from build123d import *

# Parameters (mm, degrees)
MODEL_R         = 19.166698656
MODEL_R_2       = 18.385271544
MODEL_R_3       = 16.640009412
MODEL_R_4       = 16.752801617
MODEL_W         = 2
MODEL_H         = 10
MODEL_W_2       = 2.0625
MODEL_W_3       = 5
MODEL_H_2       = 5
EXTRUDE_1_DEPTH = 1.5


with BuildPart() as part:
    # Model → 凸台-拉伸1 (new body)
    with BuildSketch(Plane.XY):
        Polygon((331.008501053, -12.681071835), (341.616416104, -12.681071835), (341.616416104, -14.681071835), (346.616416104, -14.681071835), (346.616416104, -12.681071835), (359.731458438, -12.681071835), (359.731458438, -14.681071835), (364.731458438, -14.681071835), (364.731458438, -12.681071835), (389.285051542, -12.681071835), (389.285051542, -14.681071835), (394.285051542, -14.681071835), (394.285051542, -12.681071835), (438.527315214, -12.681071835), (438.527315214, -13.681071835), (443.527315214, -13.681071835), (443.527315214, -12.681071835), (466.595113664, -12.681071835), (466.595113664, -13.681071835), (471.595113664, -13.681071835), (471.595113664, -12.681071835), (509.543834164, -12.681071835), (509.543834164, -13.681071835), (514.543834164, -13.681071835), (514.543834164, -12.681071835), (534.941100783, -12.681071835), (534.941100783, -13.681071835), (539.941100783, -13.681071835), (539.941100783, -12.681071835), (567.393171936, -12.681071835), (567.393171936, -13.681071835), (572.393171936, -13.681071835), (572.393171936, -12.681071835), (590.909160047, -12.681071835), (590.909160047, -13.681071835), (595.909160047, -13.681071835), (595.909160047, -12.681071835), (621.009616189, -12.681071835), (621.009616189, -14.681071835), (626.009616189, -14.681071835), (626.009616189, -12.681071835), (639.352091775, -12.681071835), (639.352091775, -14.681071835), (644.352091775, -14.681071835), (644.352091775, -12.681071835), (662.203652971, -12.681071835), (662.203652971, -14.681071835), (667.203652971, -14.681071835), (667.203652971, -12.681071835), (673.375169904, -12.681071835), (673.375169904, 40.318928165), (667.203652971, 40.318928165), (667.203652971, 41.318928165), (662.203652971, 41.318928165), (662.203652971, 40.318928165), (619.461197001, 40.318928165), (618.879989346, 40.463263521), (612.469969479, 41.955284735), (606.036780234, 43.352226087), (599.689619006, 44.633304674), (593.327411645, 45.82195159), (586.94928996, 46.921207599), (580.557470145, 47.935980702), (574.151952199, 48.866270901), (567.734908698, 49.715987149), (561.30547145, 50.48817021), (554.907598578, 51.180900831), (548.503413488, 51.797834645), (542.093915228, 52.338928034), (535.680059227, 52.803138329), (529.259803769, 53.18955372), (522.834147903, 53.498130589), (516.404003437, 53.72682722), (509.962377034, 53.875948948), (503.521170035, 53.942974245), (497.0802952, 53.925905013), (490.639752529, 53.824741253), (488.943859674, 53.774868005), (488.943859674, 48.550761193), (490.943859674, 48.550761193), (490.943859674, 38.550761193), (488.943859674, 38.550761193), (488.943859674, 44.701347368), (483.943859674, 44.701347368), (483.943859674, 38.550761193), (481.943859674, 38.550761193), (481.943859674, 48.550761193), (483.943859674, 48.550761193), (483.943859674, 53.624339658), (477.764179108, 53.358922521), (471.328973881, 52.990271357), (464.822470484, 52.524637869), (458.325635443, 51.959487936), (451.839336947, 51.291780793), (445.366397665, 50.51738939), (438.908510356, 49.62923315), (432.467542259, 48.62422769), (426.046316041, 47.498245959), (422.774988305, 46.874345456), (419.510213514, 46.217127406), (416.253034336, 45.527547239), (413.004318963, 44.80256419), (409.762156535, 44.044263594), (406.528457911, 43.250560117), (403.303179471, 42.420454711), (400.000268013, 41.531679768), (396.709598454, 40.602332225), (395.753608128, 40.318928165), (364.731458438, 40.318928165), (364.731458438, 41.318928165), (359.731458438, 41.318928165), (359.731458438, 40.318928165), (346.616416104, 40.318928165), (346.616416104, 41.318928165), (341.616416104, 41.318928165), (341.616416104, 40.318928165), (331.008501053, 40.318928165), align=None)
        with Locations((453.628632303, 20.416282665)):
            Circle(MODEL_R, mode=Mode.SUBTRACT)
        with Locations((517.796175226, 21.864038252)):
            Circle(MODEL_R_2, mode=Mode.SUBTRACT)
        with Locations((576.99591729, 16.073011283)):
            Circle(MODEL_R_3, mode=Mode.SUBTRACT)
        with Locations((378.89019282, 16.048912753)):
            Circle(MODEL_R_4, mode=Mode.SUBTRACT)
        Polygon((334.054616565, 0.346826696), (335.34950157, 3.052981316), (338.055656189, 1.758096311), (336.760771185, -0.948058308), align=None, mode=Mode.SUBTRACT)
        Polygon((488.943859674, 7.212935553), (483.943859674, 7.212935553), (483.943859674, 3.001809248), (481.943859674, 3.001809248), (481.943859674, -6.998190752), (483.943859674, -6.998190752), (483.943859674, -1.850844057), (488.943859674, -1.850844057), (488.943859674, -6.998190752), (490.943859674, -6.998190752), (490.943859674, 3.001809248), (488.943859674, 3.001809248), align=None, mode=Mode.SUBTRACT)
        with Locations((418.104897365, 1.876528165)):
            Rectangle(MODEL_W, MODEL_H, mode=Mode.SUBTRACT)
        with Locations((547.437658193, 3.401778165)):
            Rectangle(MODEL_W, MODEL_H, mode=Mode.SUBTRACT)
        with Locations((603.344317775, 1.378728165)):
            Rectangle(MODEL_W_2, MODEL_H, mode=Mode.SUBTRACT)
        with Locations((345.447391947, 12.318928165)):
            Rectangle(MODEL_W, MODEL_H, mode=Mode.SUBTRACT)
        with Locations((418.104897365, 26.426650996)):
            Rectangle(MODEL_W, MODEL_H, mode=Mode.SUBTRACT)
        with Locations((547.437658193, 26.823552615)):
            Rectangle(MODEL_W, MODEL_H, mode=Mode.SUBTRACT)
        with Locations((603.313067775, 26.823552615)):
            Rectangle(MODEL_W, MODEL_H, mode=Mode.SUBTRACT)
        with Locations((661.824145294, 25.818928165)):
            Rectangle(MODEL_W, MODEL_H, mode=Mode.SUBTRACT)
        with Locations((661.824145294, -1.181071835)):
            Rectangle(MODEL_W, MODEL_H, mode=Mode.SUBTRACT)
        with Locations((646.443859674, 31.16888081)):
            Rectangle(MODEL_W_3, MODEL_H_2, mode=Mode.SUBTRACT)
        with Locations((646.443859674, 0.259792132)):
            Rectangle(MODEL_W_3, MODEL_H_2, mode=Mode.SUBTRACT)
    extrude(amount=EXTRUDE_1_DEPTH)


solid = part.part
Model file for the job. Use its own axes, mm. Round coordinates to 2 decimals unless told otherwise and drop trailing zeros. Loops run counter-clockwise (first coordinate to the right, second up) from the corner with the lowest first, then second, coordinate; pieces in that order, holes last. Notation, with made-up numbers: M 89,-35.5 L 135,-35.5 A29 cw 135,-6.5 Z; hole C 71,61 d8. An arc over 180 degrees is marked long. One line per question, with ' | ' between items.
1) Band-saw the part on A-A (y = 12). Give the cut face in (x, z), then the cut area to 3 significant figures.
Solved:
outline: M 331.01,0 L 344.45,0 L 344.45,1.5 L 331.01,1.5 Z; M 346.45,0 L 362.63,0 L 362.63,1.5 L 346.45,1.5 Z; M 395.15,0 L 436.41,0 L 436.41,1.5 L 395.15,1.5 Z; M 470.85,0 L 502.28,0 L 502.28,1.5 L 470.85,1.5 Z; M 533.31,0 L 560.86,0 L 560.86,1.5 L 533.31,1.5 Z; M 593.13,0 L 673.38,0 L 673.38,1.5 L 593.13,1.5 Z | area: 315 mm²
2) Flat gauge pins, fed straight in: pin 1 (0.8 mm diameter, centred on x = 662.5, z = 0.5, fed in from +Y); pin 2 (0.8 mm diameter, centred on x = 547, z = 1, fed in from -Y); pin 3 (0.5 mm diameter, centred on y = -13, z = 0.5, fed in from -X); pin 4 (3 mm diameter, centred on x = 582.5, y = -7, fed in from -Z). Where does each tip first touch, or does it go through?
Solved:
pin 1: stops at y = 41.32 | pin 2: stops at y = -12.68 | pin 3: stops at x = 341.62 | pin 4: stops at z = 0
3) Mould opens along Y. For faces 1 (the cylindrical face through (366.54, 27.37, 0.74)), 2 (the cylindrical face through (592.367, 9.7, 0.74)), 3 (the flat face through (500, 12, 0)) say: +Y half, -Y half, draft (parallel to the pull), parting line (faces both ways), or undercut.
Solved:
face 1: undercut | face 2: undercut | face 3: draft
4) Band-saw the part on B-B (z = 0.25). Give the number of separate pieces and of enclosed holes in the cut face, then the cut area to 3 significant figures.
Solved:
separate pieces: 1 | enclosed holes: 17 | area: 15,900 mm²
5) Drill centre lines: line 1 along X through (y, z) = (-6, 1.35); line 2 along X through (y, z) = (36, 0.5); line 3 along Y through (x, z) = (481.5, 0.6). Where is each one in solid material? Low to high.
Solved:
line 1: x = 331.01 to 481.94, 483.94 to 488.94, 490.94 to 660.82, 662.82 to 673.38 | line 2: x = 331.01 to 442.47, 464.79 to 506.04, 529.55 to 673.38 | line 3: y = -12.68 to 53.52
